from build123d import *

# Parameters (mm, degrees)
F1_DEPTH = 12.7
F3_D     = 15.875


# Not quite as in the source:
# - a length typed as a fraction of an inch, garbled in the dataset ("3 / 203.2 mm" for 3/8 in), is restored


with BuildPart() as f1:
    # F0 (on Front) → F1 (new body)
    with BuildSketch(Plane.XZ):
        Polygon((114.3, 0), (0, 197.9734073051), (-114.3, 0), align=None)
    extrude(amount=F1_DEPTH)

    # F3 (through all)
    with Locations(Plane.XZ.offset(12.7)):
        with Locations((0, 168.6440136303), (-88.9, 14.6646968374), (88.9, 14.6646968374)):
            Hole(F3_D / 2)


solid = f1.part
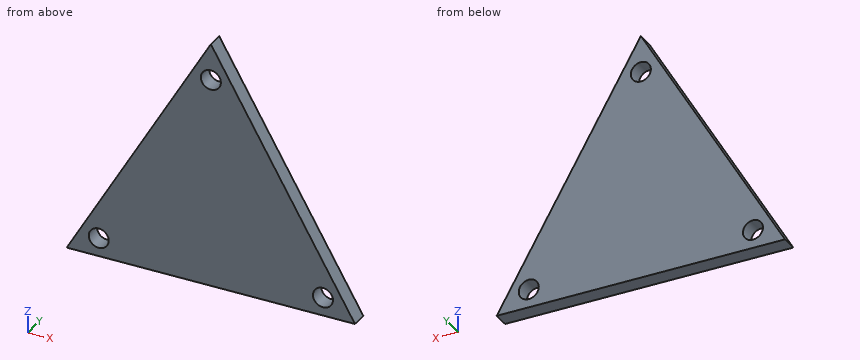
Could you check a few things on this model? Use its own coordinates, in mm. Round coordinates to 2 decimals unless told otherwise and drop trailing zeros. Order: outer loops, then holes, each group sorted by start corner. A loop starts at its lowest first (then second) coordinate and runs counter-clockwise, first axis right, second up.
Q1. I'm going to push flat-ended pins straight in: P1, Ø4, axis at y = -9.5, z = 163, coming from the -X side; P2, Ø2, axis at y = -11.5, z = 84, coming from the -X side; P3, Ø5, axis at y = -6, z = 71, coming from the +X side. Where does each tip first touch, or does it pass through?
Geometry says:
P1: stops at x = -21.35
P2: stops at x = -66.38
P3: stops at x = 74.75
Q2. Imagine slicing it at D-D, the plane z = 54. List the corners of the cut face in (x, y) for me.
Geometry says:
outline: (-83.12, -12.7) - (83.12, -12.7) - (83.12, 0) - (-83.12, 0) - close
Q3. Imagine slicing it at A-A, the plane x = 4.5. List the corners of the cut face in (y, z) for me, then the cut area to 3 significant figures.
Geometry says:
outline: (-12.7, 0) - (0, 0) - (0, 162.11) - (-12.7, 162.11) - close; (-12.7, 175.18) - (0, 175.18) - (0, 190.18) - (-12.7, 190.18) - close
area: 2,250 mm2
Q4. Please list where these lines run through material, in increasing order: probe 1 along Z at (x, y) = (0, -3); probe 2 along X at (y, z) = (-12, 18.5); probe 3 along X at (y, z) = (-2.5, 10).
Geometry says:
probe 1: z = 0 to 160.71, 176.58 to 197.97
probe 2: x = -103.62 to -95.85, -81.95 to 81.95, 95.85 to 103.62
probe 3: x = -108.53 to -95.32, -82.48 to 82.48, 95.32 to 108.53
Q5. Imagine slicing it at C-C, the plane x = 88.9. List the corners of the cut face in (y, z) for me, then the cut area to 3 significant figures.
Geometry says:
outline: (-12.7, 0) - (0, 0) - (0, 6.73) - (-12.7, 6.73) - close; (-12.7, 22.6) - (0, 22.6) - (0, 43.99) - (-12.7, 43.99) - close
area: 357 mm2
Q6. Imagine slicing it at B-B, the plane y = -3.5. List the corners of the cut face in (x, z) for me (1 decimal).
Geometry says:
outline: (-114.3, 0) - (114.3, 0) - (0, 198) - close; hole circle Ø15.9 at (-88.9, 14.7); hole circle Ø15.9 at (0, 168.6); hole circle Ø15.9 at (88.9, 14.7)
